```python
from build123d import *

# Parameters (mm, degrees)
F0_W      = 40
F0_H      = 45
F1_DEPTH  = 5
F2_R      = 1.5
F3_DEPTH  = 25
F6_DEPTH  = 25
F7_R      = 1
F8_DEPTH  = 5
F9_R      = 2.7
F10_DEPTH = 25


with BuildPart() as f1:
    # F0 (on Front) → F1 (new body)
    with BuildSketch(Plane.XZ):
        Rectangle(F0_W, F0_H)
    extrude(amount=F1_DEPTH)

    # F2 (on face) → F3 (cut)
    with BuildSketch(Plane.XZ.offset(5)):
        with Locations((16, 12.5)):
            Circle(F2_R)
        with Locations((-16, 12.5)):
            Circle(F2_R)
    extrude(amount=-F3_DEPTH, mode=Mode.SUBTRACT)

    # F5 (on face) → F6 (cut)
    with BuildSketch(Plane.XZ.offset(5)):
        Polygon((0.173205, 22.6), (-0.173205, 22.6), (0, 22.3), align=None)
    extrude(amount=-F6_DEPTH, mode=Mode.SUBTRACT)

    # F7 (on face) → F8 (cut)
    with BuildSketch(Plane.XY.offset(22.5)):
        with Locations((16, -2.5)):
            Circle(F7_R)
        with Locations((-16, -2.5)):
            Circle(F7_R)
    extrude(amount=-F8_DEPTH, mode=Mode.SUBTRACT)

    # F9 (on face) → F10 (cut)
    with BuildSketch(Plane.XZ.offset(5)):
        with Locations((0, -16.5)):
            Circle(F9_R)
    extrude(amount=-F10_DEPTH, mode=Mode.SUBTRACT)


solid = f1.part
```
Check sheet for the modelled part. Datum: model origin and axes. Units: mm. A direction names the side the tool comes from. Round coordinates to 2 decimals unless told otherwise and drop trailing zeros. Order: outer loops, then holes, each group sorted by start corner. A loop starts at its lowest first (then second) coordinate and runs counter-clockwise, first axis right, second up. Notation, with made-up numbers: (2.5, 72.5) -> (54.5, 72.5) arc R37 cw to (54.5, 108.5) -> close; hole circle Ø10 at (57.5, 65.25). An arc over 180 degrees is marked (long way). Use CSV: the item, a comma, the result in double quotes.
(1) Depth check by flat-ended pin: pin 1 (1.6 mm diameter, centred on x = 16, y = -2.5, fed in from +Z); pin 2 (4 mm diameter, centred on x = -0.5, z = -8, fed in from +Y); pin 3 (3 mm diameter, centred on x = 0, z = -16.5, fed in from -Y). Enter the tip coordinate at first touch or a pass-through.
Worked out:
pin 1,"z = 17.5"
pin 2,"y = 0"
pin 3,"through"
(2) Cross-section at B-B (y = -4.2). Record the boundary of the cut face in (x, z), and give its area (3 significant figures).
Worked out:
outline,"(-20, -22.5) -> (20, -22.5) -> (20, 22.5) -> (0.12, 22.5) -> (0, 22.3) -> (-0.12, 22.5) -> (-20, 22.5) -> close; hole circle Ø3 at (-16, 12.5); hole circle Ø5.4 at (0, -16.5); hole circle Ø3 at (16, 12.5)"
area,"1,760 mm²"
(3) Cross-section at C-C (x = -16). Record the boundary of the cut face in (y, z).
Worked out:
outline,"(-5, -22.5) -> (0, -22.5) -> (0, 11) -> (-5, 11) -> close; (-5, 14) -> (0, 14) -> (0, 22.5) -> (-1.5, 22.5) -> (-1.5, 17.5) -> (-3.5, 17.5) -> (-3.5, 22.5) -> (-5, 22.5) -> close"
(4) Tool access check on faces 4 (the face through (-16, -2, 17.5)), 5 (the face through (0, -5, 0)). Record the directions out of +Z, -Z, +X, -X, +Y, -Y that give a thin tool (end or side, any length) a straight path to the whole face; none if there is none.
Worked out:
face 4,"+Z"
face 5,"+Z, -Z, +X, -X, -Y"
(5) Draft check along Z on faces 1 (the face through (-17.5, -2.54, 12.57)), 2 (the face through (16, -2, 17.5)), 3 (the face through (-15.046, -2.2, 20.035)). Enter one of: pulls with the +Z half, pulls with the -Z half, needs draft (parallel to the pull), parting line crosses it, or undercut.
Worked out:
face 1,"undercut"
face 2,"pulls with the +Z half"
face 3,"needs draft"
(6) Cross-section at D-D (z = -16.5). Record the boundary of the cut face in (x, y).
Worked out:
outline,"(-20, -5) -> (-2.7, -5) -> (-2.7, 0) -> (-20, 0) -> close; (2.7, -5) -> (20, -5) -> (20, 0) -> (2.7, 0) -> close"
(7) Cross-section at A-A (z = 12.5). Record the boundary of the cut face in (x, y).
Worked out:
outline,"(-20, -5) -> (-17.5, -5) -> (-17.5, 0) -> (-20, 0) -> close; (-14.5, -5) -> (14.5, -5) -> (14.5, 0) -> (-14.5, 0) -> close; (17.5, -5) -> (20, -5) -> (20, 0) -> (17.5, 0) -> close"
(8) Material ranges on line 1 along Z through (x, y) = (16, -3.8); line 2 along X through (y, z) = (-0.8, 12); line 3 along Y through (x, z) = (16, 18.5), recorded low to high. Write a range as from..to.
Worked out:
line 1,"-22.5..11, 14..22.5"
line 2,"-20..-17.41, -14.59..14.59, 17.41..20"
line 3,"-5..-3.5, -1.5..0"
